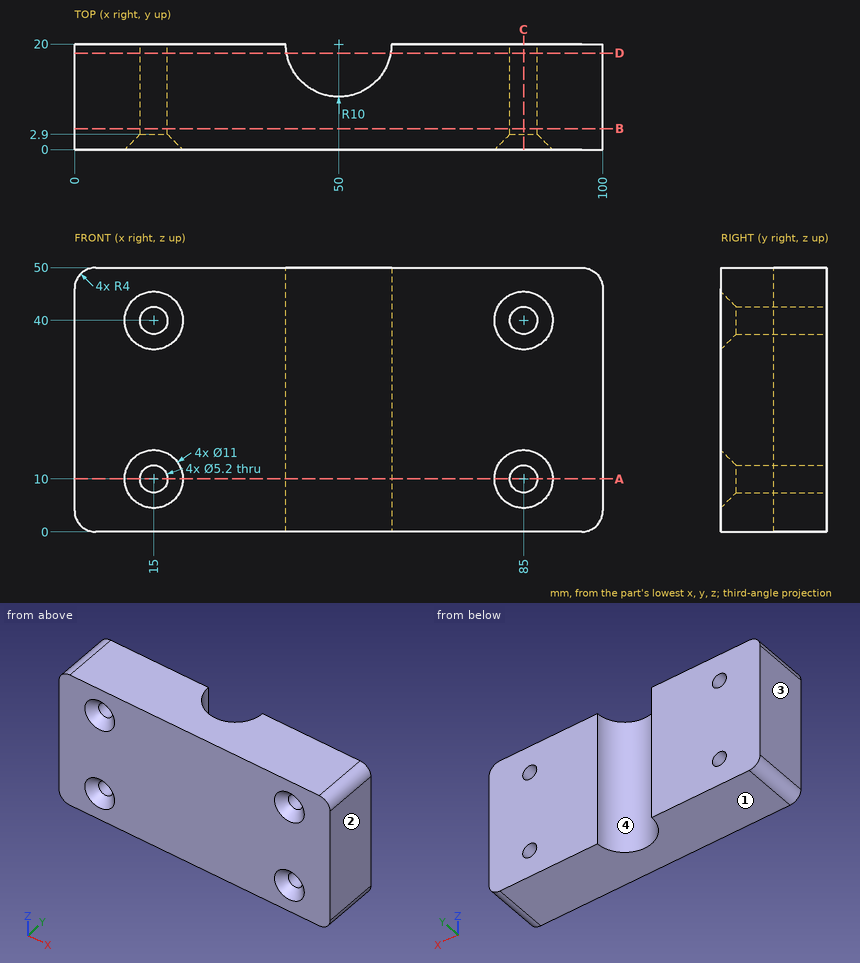
For this review, use the dimensioned drawing (mm, ordinates from the lowest corner) and the shaded views. Coordinates: 2 decimals unless noted, no trailing zeros. Order: outer loops, then holes, each group sorted by start corner. A loop starts at its lowest first (then second) coordinate and runs counter-clockwise, first axis right, second up. Notation, with made-up numbers: (66.25, -38) - (83.25, -38) arc R18 ccw to (83.25, -30) - close; hole circle Ø9 at (61, 20). An arc over 180 degrees is marked (long way). Use one line per item in the form item = value.
Q1. Consider section A-A (z = 10). Give the boundary of the cut face in (x, y), then the cut area to 3 significant figures.
Checked values:
outline = (0, 0) - (9.5, 0) - (12.4, 2.9) - (12.4, 20) - (0, 20) - close; (17.6, 2.9) - (20.5, 0) - (79.5, 0) - (82.4, 2.9) - (82.4, 20) - (60, 20) arc R10 cw to (40, 20) - (17.6, 20) - close; (87.6, 2.9) - (90.5, 0) - (100, 0) - (100, 20) - (87.6, 20) - close
area = 1,620 mm2
Q2. Consider section B-B (y = 4). Give the boundary of the cut face in (x, z).
Checked values:
outline = (0, 4) arc R4 ccw to (4, 0) - (96, 0) arc R4 ccw to (100, 4) - (100, 46) arc R4 ccw to (96, 50) - (4, 50) arc R4 ccw to (0, 46) - close; hole circle Ø5.2 at (15, 10); hole circle Ø5.2 at (15, 40); hole circle Ø5.2 at (85, 10); hole circle Ø5.2 at (85, 40)
Q3. Consider section C-C (x = 85). Give the boundary of the cut face in (y, z), then the cut area to 3 significant figures.
Checked values:
outline = (0, 0) - (20, 0) - (20, 7.4) - (2.9, 7.4) - (0, 4.5) - close; (0, 15.5) - (2.9, 12.6) - (20, 12.6) - (20, 37.4) - (2.9, 37.4) - (0, 34.5) - close; (0, 45.5) - (2.9, 42.6) - (20, 42.6) - (20, 50) - (0, 50) - close
area = 775 mm2
Q4. Draft analysis for pull direction X (two halves, no side actions). For the marked faces 1, 2, 3 and 4, state which applies: +X half, -X half, draft (parallel to the pull), parting line (faces both ways), or undercut.
Checked values:
face_1 = draft
face_2 = +X half
face_3 = -X half
face_4 = undercut
Q5. Consider section D-D (y = 18.25). Give the boundary of the cut face in (x, z), then the cut area to 3 significant figures.
Checked values:
outline = (0, 4) arc R4 ccw to (4, 0) - (40.15, 0) - (40.15, 50) - (4, 50) arc R4 ccw to (0, 46) - close; (59.85, 0) - (96, 0) arc R4 ccw to (100, 4) - (100, 46) arc R4 ccw to (96, 50) - (59.85, 50) - close; hole circle Ø5.2 at (15, 10); hole circle Ø5.2 at (15, 40); hole circle Ø5.2 at (85, 10); hole circle Ø5.2 at (85, 40)
area = 3,920 mm2
Q6. For probe 1 along Z at (x, y) = (15, 13.75); probe 2 along X at (y, z) = (8, 10); probe 3 along X at (y, z) = (6.5, 38.5), list the stretches that pass through material, from the lowest coordinate up. Write a range as from..to.
Checked values:
probe_1 = 0..7.4, 12.6..37.4, 42.6..50
probe_2 = 0..12.4, 17.6..82.4, 87.6..100
probe_3 = 0..12.88, 17.12..82.88, 87.12..100
Q7. For P1, Ø4.5, axis at x = 15, z = 40, coming from the +Y side; P2, Ø10, axis at x = 47, z = 34.5, coming from the +Y side; P3, Ø3, axis at x = 17, z = 39.5, coming from the -Y side, all flat-tipped, find the tip position at first contact; note any pin that passes through.
Checked values:
P1 = through
P2 = 14
P3 = 1.94
